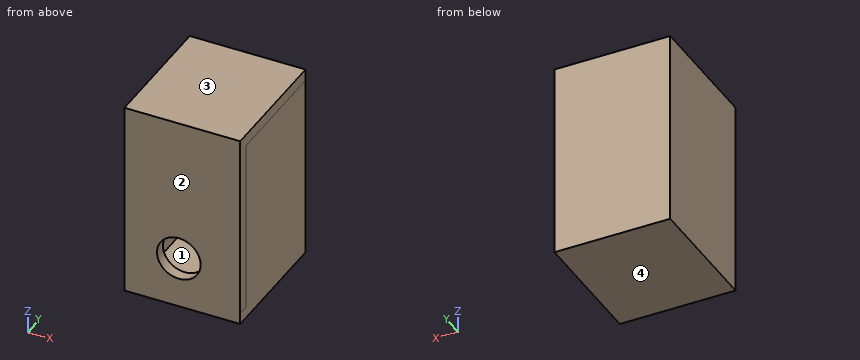
```python
from build123d import *

# Parameters (mm, degrees)
F0_W      = 200
F0_H      = 300
F1_DEPTH  = 1.5
F2_W      = 20
F2_H      = 300
F3_DEPTH  = 200
F4_W      = 20
F4_H      = 300
F5_DEPTH  = 200
F6_W      = 200.020596385
F6_H      = 300
F7_DEPTH  = 20
F8_W      = 200.020596385
F8_H      = 220
F9_DEPTH  = 20
F10_W     = 200
F10_H     = 220
F9_FACE_W = 200.020596385
F9_FACE_H = 220
F11_DEPTH = 20
F12_R     = 37.7291008544
F13_DEPTH = 92


with BuildPart() as f1:
    # F0 (on Front) → F1 (new body)
    with BuildSketch(Plane.XZ):
        with Locations((100, 150)):
            Rectangle(F0_W, F0_H)
    extrude(amount=F1_DEPTH)

    # F2 (on Front) → F3 (join)
    with BuildSketch(Plane.XZ):
        with Locations((10, 150)):
            Rectangle(F2_W, F2_H)
    extrude(amount=F3_DEPTH)

    # F4 (on face) → F5 (join)
    with BuildSketch(Plane.XZ.offset(1.5)):
        with Locations((190, 150)):
            Rectangle(F4_W, F4_H)
    extrude(amount=F5_DEPTH)

    # F6 (on face) → F7 (join)
    with BuildSketch(Plane.XZ.offset(200)):
        with Locations((100.0102981925, 150)):
            Rectangle(F6_W, F6_H)
    extrude(amount=F7_DEPTH)

    # F8 (on face) → F9 (join)
    with BuildSketch(Plane.XY.offset(300)):
        with Locations((100.0102981925, -110)):
            Rectangle(F8_W, F8_H)
    extrude(amount=F9_DEPTH)

    # F10 (on face) + F9_face (on face) → F11 (join)
    with BuildSketch(Plane(origin=(0, 0, 0), x_dir=(1, 0, 0), z_dir=(0, 0, -1))):
        with Locations((100, 110)):
            Rectangle(F10_W, F10_H)
    with BuildSketch(Plane(origin=(100.0102981925, -110, 320), x_dir=(1, 0, 0), z_dir=(0, 0, 1))):
        Rectangle(F9_FACE_W, F9_FACE_H)
    extrude(amount=F11_DEPTH, dir=(0, 0, -1))

    # F12 (on face) → F13 (cut)
    with BuildSketch(Plane.XZ.offset(220)):
        with Locations((93.9410999417, 68.8626393676)):
            Circle(F12_R)
    extrude(amount=-F13_DEPTH, mode=Mode.SUBTRACT)


solid = f1.part
```
Check sheet for the modelled part. Datum: model origin and axes. Units: mm. Face numbers are marked on the shaded views. Give positions to 0.01 mm unless a question says otherwise; leave off trailing zeros. Loops run counter-clockwise (first coordinate to the right, second up) from the corner with the lowest first, then second, coordinate; pieces in that order, holes last. Notation, with made-up numbers: (-28.5, -27.5) - (2.5, -27.5) arc R17 ccw to (2.5, -11.5) - close; hole circle Ø7 at (18, 41). An arc over 180 degrees is marked (long way). One line per question, with ' | ' between items. Start each with the question number.
1. Cross-section at C-C, the plane x = 171.5. Enter the section's corners in (y, z).
2. Gauge pin test, flat end, axial feed: pin 1 Ø10 at (y, z) = (-104.5, 125.5) entering from +X. Record the tip position at first contact, or that the pin passes through.
3. Draft check along Z on the marked faces 1, 2, 3 and 4. Enter one of: released by +Z, released by -Z, zero draft, split by the parting line, or undercut.
4. Material ranges on line 1 along Y through (x, z) = (171, 128.5); line 2 along X through (y, z) = (-131.5, 4.5); line 3 along Z through (x, y) = (100, -75), recorded low to high. Write a range as [from, to].
Check result:
1) outline: (-220, -20) - (0, -20) - (0, 320) - (-220, 320) - close; hole (-200, 0) - (-1.5, 0) - (-1.5, 300) - (-200, 300) - close
2) pin 1: stops at x = 200
3) face 1: undercut | face 2: zero draft | face 3: released by +Z | face 4: released by -Z
4) line 1: y = [-220, -200], [-1.5, 0] | line 2: x = [0, 20], [180, 200] | line 3: z = [-20, 0], [300, 320]
